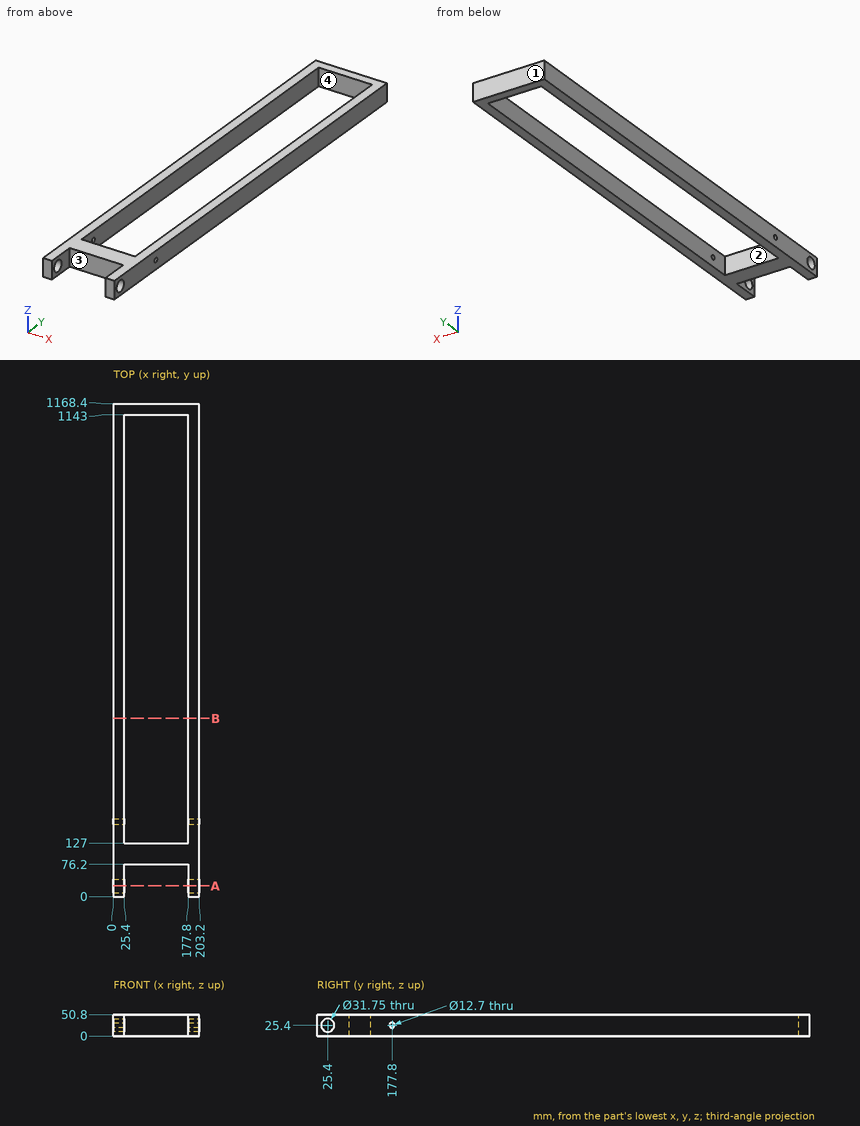
Can you work these out from the drawing? Everything is in mm from the part's minimum corner. A direction names the side the tool comes from. Give positions to 0.01 mm unless a question says otherwise; leave off trailing zeros. Loops run counter-clockwise (first coordinate to the right, second up) from the corner with the lowest first, then second, coordinate; pieces in that order, holes last. Notation, with made-up numbers: (2, 67) -> (18, 67) arc R18 cw to (18, 87) -> close; hole circle Ø8 at (34.25, -25.75). An arc over 180 degrees is marked (long way). Return JSON: item names as keys, results as strings.
Item 1: We'd pull the mould along X, two halves only. Please class the marked faces 1 and 2: +X half, -X half, draft (parallel to the pull), parting line (faces both ways), or undercut.
Geometry results:
{"face 1": "draft", "face 2": "undercut"}
Item 2: Which directions (+Z, -Z, +X, -X, +Y, -Y) give clear straight access to the entire face, cutting with the end or side of a thin tool? Please do the marked faces 3 and 4.
Geometry results:
{"face 3": "+Z, -Z, -Y", "face 4": "+Z, -Z"}
Item 3: If we section it at A-A on y = 25.4: List the corners of the cut face in (x, z) for me (3 decimals).
Geometry results:
{"outline": "(0, 0) -> (25.4, 0) -> (25.4, 9.525) -> (0, 9.525) -> close; (0, 41.275) -> (25.4, 41.275) -> (25.4, 50.8) -> (0, 50.8) -> close; (177.8, 0) -> (203.2, 0) -> (203.2, 9.525) -> (177.8, 9.525) -> close; (177.8, 41.275) -> (203.2, 41.275) -> (203.2, 50.8) -> (177.8, 50.8) -> close"}
Item 4: If we section it at B-B on y = 422.5: List the corners of the cut face in (x, z) for me.
Geometry results:
{"outline": "(0, 0) -> (25.4, 0) -> (25.4, 50.8) -> (0, 50.8) -> close; (177.8, 0) -> (203.2, 0) -> (203.2, 50.8) -> (177.8, 50.8) -> close"}
Item 5: I need wall thicknesses on L1, parallel to Y at x = 10, z = 25; L2, parallel to X at y = 807, z = 19.5; L3, parallel to Z at x = 189, y = 177. Which ranges of each line are inside material? Lowest first, please. Write a range as from..to.
Geometry results:
{"L1": "y = 0..9.53, 41.27..171.46, 184.14..1168.4", "L2": "x = 0..25.4, 177.8..203.2", "L3": "z = 0..19.1, 31.7..50.8"}
